CAD build for the part. Positions are in the model's coordinates, mm. A direction names the side the tool comes from. Round coordinates to 2 decimals unless told otherwise and drop trailing zeros. Loops run counter-clockwise (first coordinate to the right, second up) from the corner with the lowest first, then second, coordinate; pieces in that order, holes last.
Autodesk Fusion 360 part; units mm, degrees
sketch "Sketch10" plane through (0, 0, 0) normal (0, 0, 1) x (1, 0, 0)
  line L0 (0, 0) -> (45.72, 0)
  arc A0 (48.26, -2.54) -> (45.72, 0) centre (45.72, -2.54) ccw
  line L1 (45.72, -2.54) -> (48.26, -2.54) construction
  line L2 (45.72, -2.54) -> (45.72, 0) construction
  line L3 (48.26, -2.54) -> (48.26, -42.4361)
  arc A1 (48.26, -2.54) -> (45.72, 0) centre (45.72, -2.54) ccw
  arc A2 (45.72, -44.9761) -> (48.26, -42.4361) centre (45.72, -42.4361) ccw
  line L4 (0, -42.4361) -> (-2.54, -42.4361) construction
  line L5 (45.72, -44.9761) -> (0, -44.9761)
  arc A3 (-2.54, -42.4361) -> (0, -44.9761) centre (0, -42.4361) ccw
  arc A4 (-2.54, -42.4361) -> (0, -44.9761) centre (0, -42.4361) ccw
  line L6 (0, -42.4361) -> (0, -44.9761) construction
  arc A5 (0, 0) -> (-2.54, -2.54) centre (0, -2.54) ccw
  line L7 (-2.54, -42.4361) -> (-2.54, -2.54)
  point P0 (45.72, -44.9761)
  dimension "d5" = 45.72
  dimension "d7" = 2.54
  dimension "d8" = 90
  dimension "d9" = 39.8961
  dimension "d10" = 2.54
  dimension "d11" = 2.54
  dimension "d12" = 45.72
  dimension "d13" = 2.54
  dimension "d14" = 90
  dimension "d15" = 39.8961
  dimension "d16" = 2.54
  dimension "d17" = 2.54
extrude "Extrude3" add sketch "Sketch10" along normal blind 4
sketch "Sketch11" plane through (0, 0, 4) normal (0, 0, 1) x (-1, 0, 0)
  arc A0 (-45.72, 44.9761) -> (-48.26, 42.4361) centre (-45.72, 42.4361) ccw
  line L0 (-48.26, 42.4361) -> (-48.26, 2.54)
  arc A1 (-48.26, 2.54) -> (-45.72, 0) centre (-45.72, 2.54) ccw
  line L1 (-45.72, 0) -> (0, 0)
  arc A2 (0, 0) -> (2.54, 2.54) centre (0, 2.54) ccw
  line L2 (2.54, 2.54) -> (2.54, 42.4361)
  arc A3 (2.54, 42.4361) -> (0, 44.9761) centre (0, 42.4361) ccw
  line L3 (0, 44.9761) -> (-45.72, 44.9761)
  circle A4 centre (-1.778, 4.318) radius 1.75
  dimension "d22" = 3.5
extrude "Extrude4" cut sketch "Sketch11" against normal blind 4 contours A4
sketch "Sketch12" plane through (0, 0, 4) normal (0, 0, 1) x (-1, 0, 0)
  circle A0 centre (-1.778, 4.318) radius 1.75
  arc A1 (-45.72, 44.9761) -> (-48.26, 42.4361) centre (-45.72, 42.4361) ccw
  line L0 (-48.26, 42.4361) -> (-48.26, 2.54)
  arc A2 (-48.26, 2.54) -> (-45.72, 0) centre (-45.72, 2.54) ccw
  line L1 (-45.72, 0) -> (0, 0)
  arc A3 (0, 0) -> (2.54, 2.54) centre (0, 2.54) ccw
  line L2 (2.54, 2.54) -> (2.54, 42.4361)
  arc A4 (2.54, 42.4361) -> (0, 44.9761) centre (0, 42.4361) ccw
  line L3 (0, 44.9761) -> (-45.72, 44.9761)
  circle A5 centre (-43.942, 4.318) radius 1.75
  dimension "d27" = 3.5
extrude "Extrude5" cut sketch "Sketch12" against normal blind 4 contours A5
sketch "Sketch13" plane through (0, 0, 4) normal (0, 0, 1) x (-1, 0, 0)
  circle A0 centre (-43.942, 4.318) radius 1.75
  circle A1 centre (-1.778, 4.318) radius 1.75
  arc A2 (-45.72, 44.9761) -> (-48.26, 42.4361) centre (-45.72, 42.4361) ccw
  line L0 (-48.26, 42.4361) -> (-48.26, 2.54)
  arc A3 (-48.26, 2.54) -> (-45.72, 0) centre (-45.72, 2.54) ccw
  line L1 (-45.72, 0) -> (0, 0)
  arc A4 (0, 0) -> (2.54, 2.54) centre (0, 2.54) ccw
  line L2 (2.54, 2.54) -> (2.54, 42.4361)
  arc A5 (2.54, 42.4361) -> (0, 44.9761) centre (0, 42.4361) ccw
  line L3 (0, 44.9761) -> (-45.72, 44.9761)
  circle A6 centre (-1.778, 40.6581) radius 1.75
  dimension "d32" = 3.5
extrude "Extrude6" cut sketch "Sketch13" against normal blind 4 contours A6
sketch "Sketch14" plane through (0, 0, 4) normal (0, 0, 1) x (-1, 0, 0)
  circle A0 centre (-1.778, 40.6581) radius 1.75
  circle A1 centre (-43.942, 4.318) radius 1.75
  circle A2 centre (-1.778, 4.318) radius 1.75
  arc A3 (-45.72, 44.9761) -> (-48.26, 42.4361) centre (-45.72, 42.4361) ccw
  line L0 (-48.26, 42.4361) -> (-48.26, 2.54)
  arc A4 (-48.26, 2.54) -> (-45.72, 0) centre (-45.72, 2.54) ccw
  line L1 (-45.72, 0) -> (0, 0)
  arc A5 (0, 0) -> (2.54, 2.54) centre (0, 2.54) ccw
  line L2 (2.54, 2.54) -> (2.54, 42.4361)
  arc A6 (2.54, 42.4361) -> (0, 44.9761) centre (0, 42.4361) ccw
  line L3 (0, 44.9761) -> (-45.72, 44.9761)
  circle A7 centre (-43.942, 40.6581) radius 1.75
  dimension "d37" = 3.5
extrude "Extrude7" cut sketch "Sketch14" against normal blind 4 contours A7
sketch "Sketch15" plane through (0, 0, 4) normal (0, 0, 1) x (-1, 0, 0)
  circle A0 centre (-43.942, 40.6581) radius 1.75
  circle A1 centre (-1.778, 40.6581) radius 1.75
  circle A2 centre (-43.942, 4.318) radius 1.75
  circle A3 centre (-1.778, 4.318) radius 1.75
  arc A4 (-45.72, 44.9761) -> (-48.26, 42.4361) centre (-45.72, 42.4361) ccw
  line L0 (-48.26, 42.4361) -> (-48.26, 2.54)
  arc A5 (-48.26, 2.54) -> (-45.72, 0) centre (-45.72, 2.54) ccw
  line L1 (-45.72, 0) -> (0, 0)
  arc A6 (0, 0) -> (2.54, 2.54) centre (0, 2.54) ccw
  line L2 (2.54, 2.54) -> (2.54, 42.4361)
  arc A7 (2.54, 42.4361) -> (0, 44.9761) centre (0, 42.4361) ccw
  line L3 (0, 44.9761) -> (-45.72, 44.9761)
  line L4 (-4.96, 7.5) -> (-40.76, 7.5)
  line L5 (-40.76, 7.5) -> (-40.76, 37.4761)
  line L6 (-40.76, 37.4761) -> (-4.96, 37.4761)
  line L7 (-4.96, 37.4761) -> (-4.96, 7.5)
extrude "Extrude8" cut sketch "Sketch15" against normal blind 2 contours L4 L5 L6 L7
Item 1: Flat gauge pins, fed straight in: P1, Ø3, axis at x = 40, y = -39, coming from the -Z side; P2, Ø4, axis at x = 22.5, y = -31.5, coming from the +Z side. Where does each tip first touch, or does it go through?
Verdict:
P1: stops at z = 0
P2: stops at z = 2
Item 2: Cut at B-B (z = 3.45). List the corners of the cut face in (x, y), plus the area to 3 significant figures.
Verdict:
outline: (-2.54, -42.44) arc R2.54 ccw to (0, -44.98) - (45.72, -44.98) arc R2.54 ccw to (48.26, -42.44) - (48.26, -2.54) arc R2.54 ccw to (45.72, 0) - (0, 0) arc R2.54 ccw to (-2.54, -2.54) - close; hole circle Ø3.5 at (1.78, -40.66); hole circle Ø3.5 at (1.78, -4.32); hole (4.96, -37.48) - (40.76, -37.48) - (40.76, -7.5) - (4.96, -7.5) - close; hole circle Ø3.5 at (43.94, -40.66); hole circle Ø3.5 at (43.94, -4.32)
area: 1,170 mm2
Item 3: 3-axis set-ups, long thin cutter, end or side, ignore diameter. For faces 5 (the cylindrical face through (-2, -44, 2)), 6 (the flat face through (4.96, -23, 3)): which of +Z, -Z, +X, -X, +Y, -Y reach the whole face in a straight line?
Verdict:
face 5: +Z, -Z, -X, -Y
face 6: +Z
Item 4: Mould opens along Y. For faces 1 (the flat face through (23, 0, 2)), 2 (the flat face through (23, -44.976, 2)), 3 (the flat face through (-2.54, -23, 2)), 4 (the cylindrical face through (42.27, -41.18, 2.03)) say: released by +Y, released by -Y, zero draft, split by the parting line, or undercut.
Verdict:
face 1: released by +Y
face 2: released by -Y
face 3: zero draft
face 4: undercut
Item 5: Cut at C-C (x = 2). List the corners of the cut face in (y, z).
Verdict:
outline: (-44.98, 0) - (-42.39, 0) - (-42.39, 4) - (-44.98, 4) - close; (-38.92, 0) - (-6.05, 0) - (-6.05, 4) - (-38.92, 4) - close; (-2.58, 0) - (0, 0) - (0, 4) - (-2.58, 4) - close
Item 6: Cut at A-A (y = -34.5). List the corners of the cut face in (x, z), plus the area to 3 significant figures.
Verdict:
outline: (-2.54, 0) - (48.26, 0) - (48.26, 4) - (40.76, 4) - (40.76, 2) - (4.96, 2) - (4.96, 4) - (-2.54, 4) - close
area: 132 mm2
Item 7: Cut at D-D (y = -5.5). List the corners of the cut face in (x, z).
Verdict:
outline: (-2.54, 0) - (0.49, 0) - (0.49, 4) - (-2.54, 4) - close; (3.07, 0) - (42.65, 0) - (42.65, 4) - (3.07, 4) - close; (45.23, 0) - (48.26, 0) - (48.26, 4) - (45.23, 4) - close
Item 8: Wall check: L1, parallel to Y at x = 44.5, z = 1; L2, parallel to Y at x = 0.5, z = 2.3; L3, parallel to X at y = -29.5, z = 2.5. Give the ranges that are in metal, low to high.
Verdict:
L1: y = -44.98 to -42.32, -39 to -5.98, -2.66 to 0
L2: y = -44.98 to -41.85, -39.46 to -5.51, -3.12 to 0
L3: x = -2.54 to 4.96, 40.76 to 48.26
